```python
from build123d import *

# Parameters (mm, degrees)
F0_R     = 6
F1_DEPTH = 10
F4_R     = 3.75
F5_DEPTH = 9
F6_R     = 2
F7_DEPTH = 3.5
F11_SIZE = 1.2


# Not quite as in the source:
# - a fillet or chamfer that OpenCascade refuses, or shapes differently, is made with other operations: its cross-section is extruded or revolved along the edge and cut away or added


with BuildPart() as f1:
    # F0 (on Top) → F1 (new body)
    with BuildSketch(Plane.XY):
        Circle(F0_R)
    extrude(amount=F1_DEPTH)

    # F2 (on Right) → F3 (revolve)
    with BuildSketch(Plane.YZ):
        Polygon((9, 0), (6, 4), (6, 0), align=None)
    revolve(axis=Axis((0, 0, 0), (0, 0, 1)))

    # F4 (on face) → F5 (cut)
    with BuildSketch(Plane(origin=(0, 0, 0), x_dir=(1, 0, 0), z_dir=(0, 0, -1))):
        Circle(F4_R)
    extrude(amount=-F5_DEPTH, mode=Mode.SUBTRACT)

    # F6 (on face) → F7 (cut)
    with BuildSketch(Plane(origin=(0, 0, 9), x_dir=(1, 0, 0), z_dir=(0, 0, -1))):
        Circle(F6_R)
    extrude(amount=-F7_DEPTH, mode=Mode.SUBTRACT)

    # F8 (on Front) → F9 (revolve, cut)
    with BuildSketch(Plane.XZ):
        Polygon((6, 4), (6, 10), (5.6855533243, 4), align=None)
    revolve(axis=Axis((0, 0, 10), (0, 0, 1)), mode=Mode.SUBTRACT)

    # F10: fillet of radius 5.08 on 1 edges, made by hand

    # F10_s1 → F10_t2 (revolve)
    with BuildSketch(Plane.XZ):
        with BuildLine():
            ThreePointArc((6, 4), (5.8107107389, 4.8763729429), (5.7784395282, 5.7723743538))
            Line((5.7784395282, 5.7723743538), (5.6769787675, 5.7776916869))
            Line((5.6769787675, 5.7776916869), (5.5840925636, 4.0053173332))
            Line((5.5840925636, 4.0053173332), (5.6855533243, 3.8984))
            ThreePointArc((5.6855533243, 3.8984), (5.8427766622, 3.8984), (5.9029704487, 3.9698698461))
            Line((5.9029704487, 3.9698698461), (6, 4))
        make_face()
    revolve(axis=Axis((0, 0, 4), (0, 0, 1)))

    # F11
    f11_edges = [f1.edges().sort_by_distance(p)[0] for p in [
        (0, -9, 0),
    ]]
    chamfer(f11_edges, length=F11_SIZE)


solid = f1.part
```
Check sheet for the modelled part. Datum: model origin and axes. Units: mm. A direction names the side the tool comes from. Round coordinates to 2 decimals unless told otherwise and drop trailing zeros. Order: outer loops, then holes, each group sorted by start corner. A loop starts at its lowest first (then second) coordinate and runs counter-clockwise, first axis right, second up. Notation, with made-up numbers: (-4.5, 2) - (52.5, 2) arc R22 ccw to (52.5, 17) - close; hole circle Ø7 at (59.5, -10). An arc over 180 degrees is marked (long way). Answer as CSV lines item,"result". Start each with the question number.
1) Tool access check on faces 1 (the face through (-3.746, -0.165, 4.437)), 2 (the face through (3, 0, 10)), 3 (the face through (5.592, 1.761, 7.387)). Record the directions out of +Z, -Z, +X, -X, +Y, -Y that give a thin tool (end or side, any length) a straight path to the whole face; none if there is none.
2) Scan lines: probe 1 along Y at (x, z) = (0, 5); probe 2 along X at (y, z) = (0, 9.7). Record each from-to range of solid material in increasing order.
3) Section check C-C (z = 8.25). Record the cut outline in (x, y), then the cut area to 3 significant figures.
4) Section check A-A (y = 0). Record the cut outline in (x, z), then the cut area to 3 significant figures.
5) Draft check along Y on faces 4 (the face through (2, 4, 0)), 5 (the face through (5.421, 2.82, 3.852)), 6 (the face through (2, 2, 9)). Enter one of: +Y half, -Y half, draft (parallel to the pull), parting line (faces both ways), or undercut.
6) Depth check by flat-ended pin: pin 1 (1.5 mm diameter, centred on y = -6, z = 1.5, fed in from +X); pin 2 (1.5 mm diameter, centred on x = 6.5, y = -1.5, fed in from -Z); pin 3 (2 mm diameter, centred on y = 1.5, z = 4.5, fed in from -X); pin 4 (3 mm diameter, centred on x = 4, z = 3, fed in from +Y). Enter the tip coordinate at first touch or a pass-through.
Determined:
1,face 1,"-Z"
1,face 2,"+Z, +X, -X, +Y, -Y"
1,face 3,"none"
2,probe 1,"-5.8 to -3.75, 3.75 to 5.8"
2,probe 2,"-5.98 to -2, 2 to 5.98"
3,outline,"circle Ø11.82 at (0, 0); hole circle Ø7.5 at (0, 0)"
3,area,"65.5 mm^2"
4,outline,"(-8.28, 0.96) - (-7.8, 0) - (-3.75, 0) - (-3.75, 9) - (-2, 9) - (-2, 10) - (-6, 10) - (-5.78, 5.77) arc R5.08 cw to (-6, 4) - close; (2, 9) - (3.75, 9) - (3.75, 0) - (7.8, 0) - (8.28, 0.96) - (6, 4) arc R5.08 cw to (5.78, 5.77) - (6, 10) - (2, 10) - close"
4,area,"57.8 mm^2"
5,face 4,"draft"
5,face 5,"parting line"
5,face 6,"undercut"
6,pin 1,"x = 6.21"
6,pin 2,"z = 0"
6,pin 3,"x = -6.23"
6,pin 4,"y = 7.01"
